from build123d import *

# Parameters (mm, degrees)
SKETCH082_W     = 445
SKETCH082_H     = 232
PAD025_DEPTH    = 3
SKETCH083_R     = 9.5
POCKET054_DEPTH = 5
FILLET010_R     = 2
POCKET055_DEPTH = 10.001
SKETCH085_R     = 6
SKETCH085_R_2   = 5
POCKET056_DEPTH = 5
SKETCH094_W     = 459.410004
SKETCH094_H     = 453.216675
POCKET063_DEPTH = 5


with BuildPart() as part:
    # Sketch082 → Pad025 (new body)
    with BuildSketch(Plane.XY):
        Rectangle(SKETCH082_W, SKETCH082_H)
    extrude(amount=PAD025_DEPTH)

    # Sketch083 (on Face6 of Pad025) → Pocket054 (cut)
    with BuildSketch(Plane.XY.offset(3)):
        with Locations((-183, 55)):
            Circle(SKETCH083_R)
        with Locations((-183, 33)):
            Circle(SKETCH083_R)
        with Locations((-183, 11)):
            Circle(SKETCH083_R)
        with Locations((-183, -11)):
            Circle(SKETCH083_R)
        with Locations((-183, -33)):
            Circle(SKETCH083_R)
        with Locations((-183, -55)):
            Circle(SKETCH083_R)
        with Locations((-164, 44)):
            Circle(SKETCH083_R)
        with Locations((-164, 22)):
            Circle(SKETCH083_R)
        with Locations((-164, 0)):
            Circle(SKETCH083_R)
        with Locations((-164, -22)):
            Circle(SKETCH083_R)
        with Locations((-164, -44)):
            Circle(SKETCH083_R)
        with Locations((-145, 55)):
            Circle(SKETCH083_R)
        with Locations((-145, 33)):
            Circle(SKETCH083_R)
        with Locations((-145, 11)):
            Circle(SKETCH083_R)
        with Locations((-145, -11)):
            Circle(SKETCH083_R)
        with Locations((-145, -33)):
            Circle(SKETCH083_R)
        with Locations((-145, -55)):
            Circle(SKETCH083_R)
        with Locations((-126, 44)):
            Circle(SKETCH083_R)
        with Locations((-126, 22)):
            Circle(SKETCH083_R)
        with Locations((-126, 0)):
            Circle(SKETCH083_R)
        with Locations((-126, -22)):
            Circle(SKETCH083_R)
        with Locations((-126, -44)):
            Circle(SKETCH083_R)
        with Locations((-107, 55)):
            Circle(SKETCH083_R)
        with Locations((-107, 33)):
            Circle(SKETCH083_R)
        with Locations((-107, 11)):
            Circle(SKETCH083_R)
        with Locations((-107, -11)):
            Circle(SKETCH083_R)
        with Locations((-107, -33)):
            Circle(SKETCH083_R)
        with Locations((-107, -55)):
            Circle(SKETCH083_R)
        with Locations((-88, -44)):
            Circle(SKETCH083_R)
        with Locations((-88, -22)):
            Circle(SKETCH083_R)
        with Locations((-88, 0)):
            Circle(SKETCH083_R)
        with Locations((-88, 22)):
            Circle(SKETCH083_R)
        with Locations((-88, 44)):
            Circle(SKETCH083_R)
        with Locations((-69, 55)):
            Circle(SKETCH083_R)
        with Locations((-69, 33)):
            Circle(SKETCH083_R)
        with Locations((-69, 11)):
            Circle(SKETCH083_R)
        with Locations((-69, -11)):
            Circle(SKETCH083_R)
        with Locations((-69, -33)):
            Circle(SKETCH083_R)
        with Locations((-50, 44)):
            Circle(SKETCH083_R)
        with Locations((-50, 22)):
            Circle(SKETCH083_R)
        with Locations((-50, 0)):
            Circle(SKETCH083_R)
        with Locations((-50, -22)):
            Circle(SKETCH083_R)
        with Locations((-50, -44)):
            Circle(SKETCH083_R)
        with Locations((-69, -55)):
            Circle(SKETCH083_R)
        with Locations((-31, 55)):
            Circle(SKETCH083_R)
        with Locations((-31, 33)):
            Circle(SKETCH083_R)
        with Locations((-31, 11)):
            Circle(SKETCH083_R)
        with Locations((-31, -11)):
            Circle(SKETCH083_R)
        with Locations((-31, -33)):
            Circle(SKETCH083_R)
        with Locations((-31, -55)):
            Circle(SKETCH083_R)
        with Locations((-12, -44)):
            Circle(SKETCH083_R)
        with Locations((-12, -22)):
            Circle(SKETCH083_R)
        with Locations((-12, 0)):
            Circle(SKETCH083_R)
        with Locations((-12, 22)):
            Circle(SKETCH083_R)
        with Locations((-12, 44)):
            Circle(SKETCH083_R)
        with Locations((7, 55)):
            Circle(SKETCH083_R)
        with Locations((7, 33)):
            Circle(SKETCH083_R)
        with Locations((7, 11)):
            Circle(SKETCH083_R)
        with Locations((7, -11)):
            Circle(SKETCH083_R)
        with Locations((7, -33)):
            Circle(SKETCH083_R)
        with Locations((7, -55)):
            Circle(SKETCH083_R)
        with Locations((26, -44)):
            Circle(SKETCH083_R)
        with Locations((26, -22)):
            Circle(SKETCH083_R)
        with Locations((26, 0)):
            Circle(SKETCH083_R)
        with Locations((26, 22)):
            Circle(SKETCH083_R)
        with Locations((26, 44)):
            Circle(SKETCH083_R)
        with Locations((45, 55)):
            Circle(SKETCH083_R)
        with Locations((45, 33)):
            Circle(SKETCH083_R)
        with Locations((45, 11)):
            Circle(SKETCH083_R)
        with Locations((45, -11)):
            Circle(SKETCH083_R)
        with Locations((64, 0)):
            Circle(SKETCH083_R)
        with Locations((64, 22)):
            Circle(SKETCH083_R)
        with Locations((64, 44)):
            Circle(SKETCH083_R)
        with Locations((45, -33)):
            Circle(SKETCH083_R)
        with Locations((45, -55)):
            Circle(SKETCH083_R)
        with Locations((64, -44)):
            Circle(SKETCH083_R)
        with Locations((64, -22)):
            Circle(SKETCH083_R)
        with Locations((83, 55)):
            Circle(SKETCH083_R)
        with Locations((83, 33)):
            Circle(SKETCH083_R)
        with Locations((83, 11)):
            Circle(SKETCH083_R)
        with Locations((83, -11)):
            Circle(SKETCH083_R)
        with Locations((83, -33)):
            Circle(SKETCH083_R)
        with Locations((83, -55)):
            Circle(SKETCH083_R)
        with Locations((102, 44)):
            Circle(SKETCH083_R)
        with Locations((102, 22)):
            Circle(SKETCH083_R)
        with Locations((102, 0)):
            Circle(SKETCH083_R)
        with Locations((102, -22)):
            Circle(SKETCH083_R)
        with Locations((102, -44)):
            Circle(SKETCH083_R)
        with Locations((121, 55)):
            Circle(SKETCH083_R)
        with Locations((121, 33)):
            Circle(SKETCH083_R)
        with Locations((121, 11)):
            Circle(SKETCH083_R)
        with Locations((121, -11)):
            Circle(SKETCH083_R)
        with Locations((121, -33)):
            Circle(SKETCH083_R)
        with Locations((121, -55)):
            Circle(SKETCH083_R)
        with Locations((140, 44)):
            Circle(SKETCH083_R)
        with Locations((140, 22)):
            Circle(SKETCH083_R)
        with Locations((140, 0)):
            Circle(SKETCH083_R)
        with Locations((140, -22)):
            Circle(SKETCH083_R)
        with Locations((140, -44)):
            Circle(SKETCH083_R)
        with Locations((159, 55)):
            Circle(SKETCH083_R)
        with Locations((159, 33)):
            Circle(SKETCH083_R)
        with Locations((159, 11)):
            Circle(SKETCH083_R)
        with Locations((159, -11)):
            Circle(SKETCH083_R)
        with Locations((159, -33)):
            Circle(SKETCH083_R)
        with Locations((159, -55)):
            Circle(SKETCH083_R)
        with Locations((-164, 66)):
            Circle(SKETCH083_R)
        with Locations((-126, 66)):
            Circle(SKETCH083_R)
        with Locations((-88, 66)):
            Circle(SKETCH083_R)
        with Locations((-50, 66)):
            Circle(SKETCH083_R)
        with Locations((-12, 66)):
            Circle(SKETCH083_R)
        with Locations((26, 66)):
            Circle(SKETCH083_R)
        with Locations((64, 66)):
            Circle(SKETCH083_R)
        with Locations((102, 66)):
            Circle(SKETCH083_R)
        with Locations((140, 66)):
            Circle(SKETCH083_R)
        with Locations((-164, -66)):
            Circle(SKETCH083_R)
        with Locations((-126, -66)):
            Circle(SKETCH083_R)
        with Locations((-88, -66)):
            Circle(SKETCH083_R)
        with Locations((-50, -66)):
            Circle(SKETCH083_R)
        with Locations((-12, -66)):
            Circle(SKETCH083_R)
        with Locations((26, -66)):
            Circle(SKETCH083_R)
        with Locations((64, -66)):
            Circle(SKETCH083_R)
        with Locations((102, -66)):
            Circle(SKETCH083_R)
        with Locations((140, -66)):
            Circle(SKETCH083_R)
        with Locations((178, 66)):
            Circle(SKETCH083_R)
        with Locations((178, 44)):
            Circle(SKETCH083_R)
        with Locations((178, 22)):
            Circle(SKETCH083_R)
        with Locations((178, 0)):
            Circle(SKETCH083_R)
        with Locations((178, -22)):
            Circle(SKETCH083_R)
        with Locations((178, -44)):
            Circle(SKETCH083_R)
        with Locations((178, -66)):
            Circle(SKETCH083_R)
    extrude(amount=-POCKET054_DEPTH, mode=Mode.SUBTRACT)

    # Fillet010
    fillet010_edges = [part.edges().sort_by_distance(p)[0] for p in [
        (-222.5, -116, 1.5),
        (222.5, -116, 1.5),
        (222.5, 116, 1.5),
        (-222.5, 116, 1.5),
    ]]
    fillet(fillet010_edges, radius=FILLET010_R)

    # Sketch084 → Pocket055 (cut, through all)
    with BuildSketch(Plane.XY.offset(10)):
        Polygon((188.873749, -62), (214.664444, -62), (214.664444, 62), (188.873749, 62), (188.873749, 11.724954), (183.462372, 4.250606), (183.462372, -4.752587), (188.873749, -11.972128), align=None)
    extrude(amount=-POCKET055_DEPTH, mode=Mode.SUBTRACT)

    # Sketch085 (on Face2 of Pocket055) → Pocket056 (cut)
    with BuildSketch(Plane(origin=(0, 0, 0), x_dir=(1, 0, 0), z_dir=(0, 0, -1))):
        with Locations((213.5, 50)):
            Circle(SKETCH085_R)
        with Locations((213.5, -50)):
            Circle(SKETCH085_R)
        with Locations((-213.5, 50)):
            Circle(SKETCH085_R)
        with Locations((-213.5, -50)):
            Circle(SKETCH085_R)
        with Locations((-163.5, 90)):
            Circle(SKETCH085_R_2)
        with Locations((-25.5, 90)):
            Circle(SKETCH085_R_2)
        with Locations((163.5, 90)):
            Circle(SKETCH085_R_2)
        with Locations((163.5, -90)):
            Circle(SKETCH085_R_2)
        with Locations((-25.5, -90)):
            Circle(SKETCH085_R_2)
        with Locations((-163.5, -90)):
            Circle(SKETCH085_R_2)
    extrude(amount=-POCKET056_DEPTH, mode=Mode.SUBTRACT)

    # Sketch094 (on Face5 of Pocket056) → Pocket063 (cut)
    with BuildSketch(Plane.XY.offset(3)):
        with Locations((-89.705002, -21.970826)):
            Rectangle(SKETCH094_W, SKETCH094_H)
    extrude(amount=-POCKET063_DEPTH, mode=Mode.SUBTRACT)


with BuildPart() as part_1:
    # Body021 placement: moved
    add(part.part.moved(Location((0, 0, -3))))


solid = part_1.part
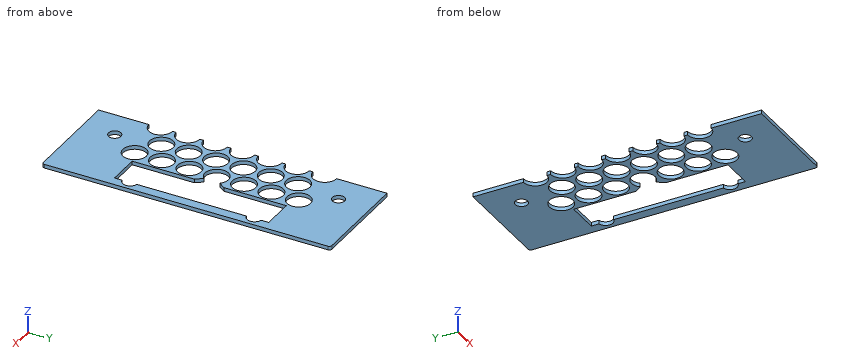
Could you check a few things on this model? Use its own coordinates, in mm. Give positions to 0.01 mm unless a question says otherwise; leave off trailing zeros. Order: outer loops, then holes, each group sorted by start corner. A loop starts at its lowest first (then second) coordinate and runs counter-clockwise, first axis right, second up.
1. Suppose I cut it at A-A (x = 205). List the corners of the cut face in (y, z) for me, plus the area to 3 significant figures.
2. I need wall thicknesses on L1, parallel to X at y = 40.5, z = -0.7; L2, parallel to X at y = -5, z = -0.65; L3, parallel to X at y = -56, z = -0.95. Which ranges of each line are inside material? Lowest first, please.
3. Suppose I cut it at D-D (z = -1.1). Give the number of separate pieces and of enclosed holes in the cut face, plus the area to 3 significant figures.
4. Will these pins go through, and if not, where does the flat tip stop? P1, Ø17, axis at x = 159, y = -11, coming from the +Z side; P2, Ø1, axis at y = -41, z = -1, coming from the -X side; P3, Ø1.5, axis at y = -58, z = -1.5, coming from the -X side.
5. Suppose I cut it at B-B (y = -38). List the corners of the cut face in (x, z) for me.
6. Suppose I cut it at C-C (x = 153). List the corners of the cut face in (y, z) for me, plus the area to 3 significant figures.
Solved:
1. outline: (-116, -3) - (-62, -3) - (-62, 0) - (-116, 0) - close; (62, -3) - (116, -3) - (116, 0) - (62, 0) - close
1. area: 324 mm2
2. L1: x = 148.83 to 153.17, 164.83 to 169.17, 186.83 to 188.87, 214.66 to 222.5
2. L2: x = 148.08 to 151.63, 166.37 to 169.92, 214.66 to 222.5
2. L3: x = 140 to 149.55, 168.45 to 188.87, 214.66 to 222.5
3. separate pieces: 1
3. enclosed holes: 15
3. area: 11,000 mm2
4. P1: passes through
4. P2: stops at x = 148.83
4. P3: stops at x = 143.7
5. outline: (147.37, -3) - (150.92, -3) - (150.92, 0) - (147.37, 0) - close; (167.08, -3) - (170.63, -3) - (170.63, 0) - (167.08, 0) - close; (185.37, -3) - (188.87, -3) - (188.87, 0) - (185.37, 0) - close; (214.66, -3) - (222.5, -3) - (222.5, 0) - (214.66, 0) - close
6. outline: (-116, -3) - (-62.37, -3) - (-62.37, 0) - (-116, 0) - close; (-47.63, -3) - (-40.37, -3) - (-40.37, 0) - (-47.63, 0) - close; (-25.63, -3) - (-18.37, -3) - (-18.37, 0) - (-25.63, 0) - close; (-3.63, -3) - (3.63, -3) - (3.63, 0) - (-3.63, 0) - close; (18.37, -3) - (25.63, -3) - (25.63, 0) - (18.37, 0) - close; (40.37, -3) - (47.63, -3) - (47.63, 0) - (40.37, 0) - close; (62.37, -3) - (116, -3) - (116, 0) - (62.37, 0) - close
6. area: 431 mm2
